Design review of the part built by this model. Coordinates are the model's own, in mm. A direction names the side the tool comes from. Coordinates: 2 decimals unless noted, no trailing zeros. Loops run counter-clockwise (first coordinate to the right, second up) from the corner with the lowest first, then second, coordinate; pieces in that order, holes last. Notation, with made-up numbers: (65.5, 5) - (74.5, 5) arc R17 cw to (74.5, 30) - close; hole circle Ø7 at (80, -28). An arc over 180 degrees is marked (long way). Use one line per item in the form item = value. Start each with the question number.
(1) Add section C-C (x = 4.5). State the section outline as (y, z) points.
(2) For L1, parallel to X at y = 168.5, z = 10; L2, parallel to Z at x = -13, y = 45, list the stretches that pass through material, from the lowest coordinate up.
(3) The part is to be moulded in two halves that separate along Y. For faces 4 (the face through (20, 0, 0)), 5 (the face through (20.95, 176.25, 1.21)), 6 (the face through (19.431, 195, 0)), say which applies: pulls with the +Y half, pulls with the -Y half, needs draft (parallel to the pull), parting line crosses it, or undercut.
(4) Clearance check with a flat-ended pin moving along its axis: pin 1 Ø1.5 at (y, z) = (132, 6) entering from +X. State where the tip first meets the part, or that it passes through.
(5) Add section D-D (y = 30). State the section outline as (x, z) points, plus the area to 3 significant figures.
(6) Tool access review of faces 1 (the face through (0, 192, 19.431)), 2 (the face through (20.952, 186.113, 1.793)), 3 (the face through (-0.272, 182.635, 20.952)): name each direction out of +Z, -Z, +X, -X, +Y, -Y from which nothing blocks a thin tool from reaching the whole face with its end or side.
(7) Add section B-B (z = -2.5). State the section outline as (x, y) points, plus the area to 3 significant figures.
(8) Add section A-A (y = 147). State the section outline as (x, z) points, plus the area to 3 significant figures.
```python
from build123d import *

# Parameters (mm, degrees)
SKETCH1_W           = 44.862
SKETCH1_H           = 44.862
SKETCH1_W_2         = 38.862
SKETCH1_H_2         = 38.862
BOSS_EXTRUDE1_DEPTH = 203.2
X_FACE_CUT_DEPTH    = 3
Y_FACE_DEPTH        = 3


with BuildPart() as part:
    # Sketch1 → Boss-Extrude1 (new body)
    with BuildSketch(Plane(origin=(0, 0, 0), x_dir=(1, 0, 0), z_dir=(0, 1, 0))):
        Rectangle(SKETCH1_W, SKETCH1_H)
        Rectangle(SKETCH1_W_2, SKETCH1_H_2, mode=Mode.SUBTRACT)
    extrude(amount=BOSS_EXTRUDE1_DEPTH)

    # Sketch3 → X Face Cut (cut)
    with BuildSketch(Plane(origin=(22.431, 0, 0), x_dir=(0, 0, -1), z_dir=(1, 0, 0))):
        Polygon((-22.431, 190.5), (19.431, 181.601957215), (19.431, 171.864163049), (-22.431, 180.762205834), align=None)
        Polygon((-22.431, 126.160248619), (19.431, 117.262205834), (19.431, 127), (-22.431, 135.898042785), align=None)
    extrude(amount=-X_FACE_CUT_DEPTH, mode=Mode.SUBTRACT)

    # Sketch4 → Y Face (cut)
    with BuildSketch(Plane.XY.offset(22.431)):
        Polygon((22.431, 180.762205834), (-19.431, 165.525683887), (-19.431, 175.66197717), (22.431, 190.898499117), align=None)
        Polygon((19.431, 109.909043825), (-19.431, 11.252109304), (-19.431, 37.241108263), (19.431, 135.898042785), align=None)
    extrude(amount=-Y_FACE_DEPTH, mode=Mode.SUBTRACT)


solid = part.part
```
Computed values:
q1.outline = (0, -22.43) - (203.2, -22.43) - (203.2, -19.43) - (0, -19.43) - close; (0, 19.43) - (72, 19.43) - (72, 22.43) - (0, 22.43) - close; (97.99, 19.43) - (174.24, 19.43) - (174.24, 22.43) - (97.99, 22.43) - close; (184.37, 19.43) - (203.2, 19.43) - (203.2, 22.43) - (184.37, 22.43) - close
q2.L1 = -22.43 to -19.43, 19.43 to 22.43
q2.L2 = -22.43 to -19.43
q3.face_4 = pulls with the -Y half
q3.face_5 = undercut
q3.face_6 = needs draft
q4.pin_1 = 22.43
q5.outline = (-22.43, -22.43) - (22.43, -22.43) - (22.43, 22.43) - (-12.05, 22.43) - (-12.05, 19.43) - (19.43, 19.43) - (19.43, -19.43) - (-19.43, -19.43) - (-19.43, 22.43) - (-22.43, 22.43) - close
q5.area = 480 mm^2
q6.face_1 = +Y, -Y
q6.face_2 = +Z, +X
q6.face_3 = +Z
q7.outline = (-22.43, 0) - (-19.43, 0) - (-19.43, 203.2) - (-22.43, 203.2) - close; (19.43, 0) - (22.43, 0) - (22.43, 120.86) - (19.43, 120.86) - close; (19.43, 130.6) - (22.43, 130.6) - (22.43, 175.46) - (19.43, 175.46) - close; (19.43, 185.2) - (22.43, 185.2) - (22.43, 203.2) - (19.43, 203.2) - close
q7.area = 1,160 mm^2
q8.outline = (-22.43, -22.43) - (22.43, -22.43) - (22.43, 22.43) - (-22.43, 22.43) - close; hole (-19.43, -19.43) - (19.43, -19.43) - (19.43, 19.43) - (-19.43, 19.43) - close
q8.area = 502 mm^2
